from build123d import *

# Parameters (mm, degrees)
F0_W     = 30
F0_H     = 17.5
F1_DEPTH = 2
F2_R     = 1.5
F3_DEPTH = 25
F4_W     = 30
F4_H     = 2
F5_DEPTH = 3
F6_W     = 30
F6_H     = 1
F7_DEPTH = 1.5


with BuildPart() as f1:
    # F0 (on Top) → F1 (new body)
    with BuildSketch(Plane.XY):
        with Locations((-15, 8.75)):
            Rectangle(F0_W, F0_H)
    extrude(amount=F1_DEPTH)

    # F2 (on face) → F3 (cut)
    with BuildSketch(Plane.XY.offset(2)):
        with Locations((-21, 8.75)):
            Circle(F2_R)
    extrude(amount=-F3_DEPTH, mode=Mode.SUBTRACT)

    # F4 (on face) → F5 (join)
    with BuildSketch(Plane.XY.offset(2)):
        with Locations((-15, 16.5)):
            Rectangle(F4_W, F4_H)
        with Locations((-15, 1)):
            Rectangle(F4_W, F4_H)
    extrude(amount=F5_DEPTH)

    # F6 (on face) → F7 (join)
    with BuildSketch(Plane.XY.offset(2)):
        with Locations((-15, 15)):
            Rectangle(F6_W, F6_H)
        with Locations((-15, 2.5)):
            Rectangle(F6_W, F6_H)
    extrude(amount=F7_DEPTH)


solid = f1.part
Read the model definition and answer for the solid it produces. Units are mm, in the model's axes. A direction names the side the tool comes from. Give positions to 0.01 mm unless a question says otherwise; leave off trailing zeros. Write each loop counter-clockwise with the first axis right and the second up, starting at its lowest first coordinate (ties: lowest second). Pieces come first, ordered by that corner, then holes. Notation, with made-up numbers: (-28, 39.5) -> (29, 39.5) arc R12 ccw to (29, 52.5) -> close; hole circle Ø4 at (-21, -36.75). An arc over 180 degrees is marked (long way). Answer as a JSON object with one key per item and string values. Group by question number.
1) Find section B-B (x = -21). Write down the section's boundary in (y, z), and give its area (3 significant figures).
2) Each of these flat-tipped pins is pushed along its axis until it touches: P1, Ø5, axis at x = -26, y = 9.5, coming from the +Z side; P2, Ø0.8, axis at x = -22, y = 15, coming from the +Z side. Where does it stop, or does it pass through?
3) Find section A-A (z = 2.4). Write down the section's boundary in (x, y).
4) Consider L1, parallel to Y at x = -8.75, z = 4.1; L2, parallel to Y at x = -21, z = 0.6; L3, parallel to Z at x = -20.25, y = 6. Determine where each line is inside the solid, lowest interval first. Write a range as from..to.
5) Find section C-C (y = 8.75). Write down the section's boundary in (x, z), and give its area (3 significant figures).
6) Find section D-D (x = -2.5). Write down the section's boundary in (y, z), and give its area (3 significant figures).
7) The mould has two halves that part along X. Classify faces 1 (the flat face through (-30, 9, 1)), 2 (the flat face through (-15.2, 2.5, 3.5)), 3 (the cylindrical face through (-22.5, 8.8, 1)): +X half, -X half, draft (parallel to the pull), parting line (faces both ways), or undercut.
8) A tool of negligible diameter and unlimited length cuts with its end or side. For faces 4 (the flat face through (-15, 15.5, 4)), 5 (the flat face through (0, 9, 1)), from which of +Z, -Z, +X, -X, +Y, -Y can it reach the whole face along a straight path? Write none if from no direction.
Values follow:
{
 "1": {"outline": "(0, 0) -> (7.25, 0) -> (7.25, 2) -> (3, 2) -> (3, 3.5) -> (2, 3.5) -> (2, 5) -> (0, 5) -> close; (10.25, 0) -> (17.5, 0) -> (17.5, 5) -> (15.5, 5) -> (15.5, 3.5) -> (14.5, 3.5) -> (14.5, 2) -> (10.25, 2) -> close", "area": "44.0 mm2"},
 "2": {"P1": "stops at z = 2", "P2": "stops at z = 3.5"},
 "3": {"outline": "(-30, 0) -> (0, 0) -> (0, 3) -> (-30, 3) -> close; (-30, 14.5) -> (0, 14.5) -> (0, 17.5) -> (-30, 17.5) -> close"},
 "4": {"L1": "y = 0..2, 15.5..17.5", "L2": "y = 0..7.25, 10.25..17.5", "L3": "z = 0..2"},
 "5": {"outline": "(-30, 0) -> (-22.5, 0) -> (-22.5, 2) -> (-30, 2) -> close; (-19.5, 0) -> (0, 0) -> (0, 2) -> (-19.5, 2) -> close", "area": "54.0 mm2"},
 "6": {"outline": "(0, 0) -> (17.5, 0) -> (17.5, 5) -> (15.5, 5) -> (15.5, 3.5) -> (14.5, 3.5) -> (14.5, 2) -> (3, 2) -> (3, 3.5) -> (2, 3.5) -> (2, 5) -> (0, 5) -> close", "area": "50.0 mm2"},
 "7": {"face 1": "-X half", "face 2": "draft", "face 3": "undercut"},
 "8": {"face 4": "+Z, +X, -X", "face 5": "+Z, -Z, +X, +Y, -Y"}
}
